For this review, use the dimensioned drawing (mm, ordinates from the lowest corner) and the shaded views. Coordinates: 2 decimals unless noted, no trailing zeros. Write each loop counter-clockwise with the first axis right and the second up, starting at its lowest first coordinate (ties: lowest second). Pieces come first, ordered by that corner, then holes.
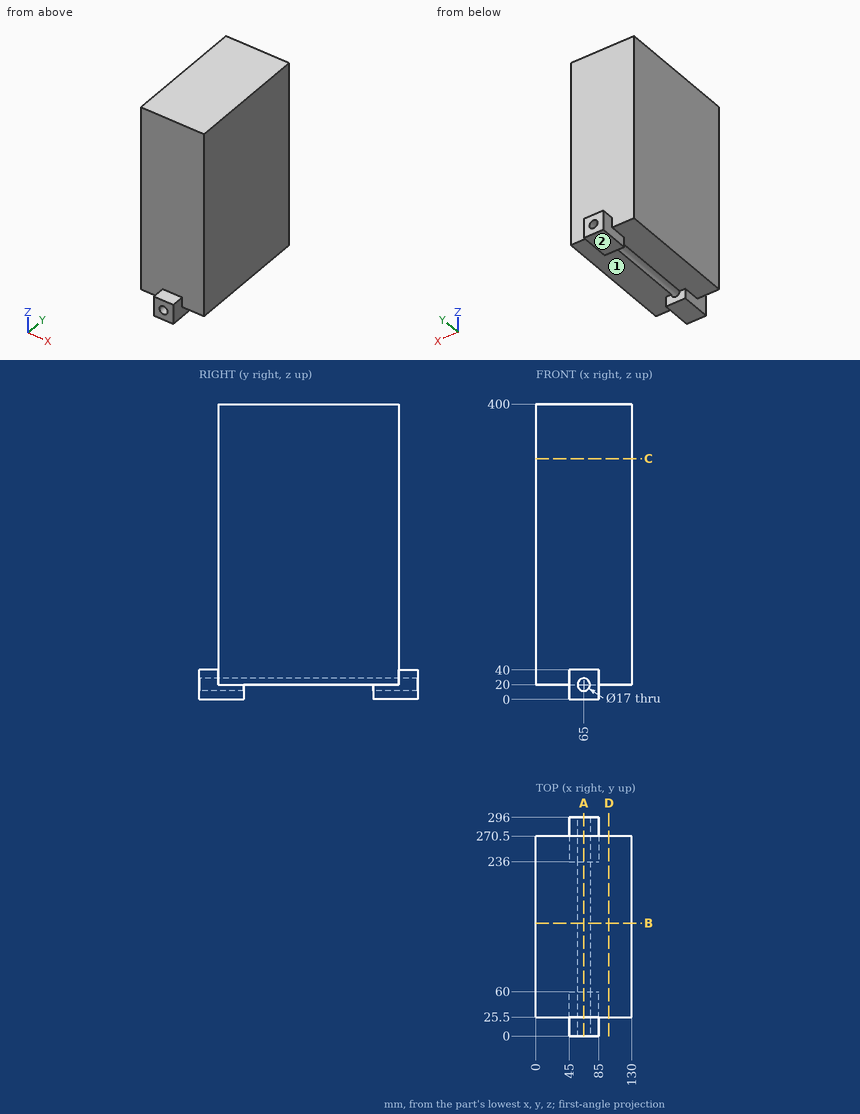
Item 1: Mouldability with a two-part tool opening along Y and no side actions: class the marked faces 1 and 2 as pulls with the +Y half, pulls with the -Y half, needs draft (parallel to the pull), parting line crosses it, or undercut.
Solved:
face 1: undercut
face 2: needs draft
Item 2: Take a section at C-C, the plane z = 326. Write out the cut boundary in (x, y), plus the area to 4 significant figures.
Solved:
outline: (0, 25.5) - (130, 25.5) - (130, 270.5) - (0, 270.5) - close
area: 31,850 mm2
Item 3: Take a section at D-D, the plane x = 99. Write out the cut boundary in (y, z).
Solved:
outline: (25.5, 20) - (270.5, 20) - (270.5, 400) - (25.5, 400) - close
Item 4: For pin 1 (1.5 mm diameter, centred on x = 100, z = 232.5, fed in from -Y); pin 2 (17 mm diameter, centred on x = 98.5, y = 208, fed in from -Z); pin 3 (13.5 mm diameter, centred on x = 65, z = 20, fed in from +Y); pin 4 (4 mm diameter, centred on x = 82.5, z = 300.5, fed in from +Y), all flat-tipped, find the tip position at first contact; note any pin that passes through.
Solved:
pin 1: stops at y = 25.5
pin 2: stops at z = 20
pin 3: passes through
pin 4: stops at y = 270.5
Item 5: Take a section at B-B, the plane y = 153. Write out the cut boundary in (x, z), plus the area to 3 significant figures.
Solved:
outline: (0, 20) - (56.5, 20) arc R8.5 cw to (73.5, 20) - (130, 20) - (130, 400) - (0, 400) - close
area: 49,300 mm2
Item 6: Take a section at A-A, the plane x = 65. Write out the cut boundary in (y, z).
Solved:
outline: (0, 0) - (60, 0) - (60, 11.5) - (0, 11.5) - close; (0, 28.5) - (296, 28.5) - (296, 40) - (270.5, 40) - (270.5, 400) - (25.5, 400) - (25.5, 40) - (0, 40) - close; (236, 0) - (296, 0) - (296, 11.5) - (236, 11.5) - close
Item 7: To check wall thickness, follow line 1 along X through (y, z) = (270, 19.5); line 2 along Y through (x, z) = (30.5, 104); line 3 along Z through (x, y) = (118, 164.5). State the ranges of each line that lie inside material, in increasing order.
Solved:
line 1: x = 45 to 56.51, 73.49 to 85
line 2: y = 25.5 to 270.5
line 3: z = 20 to 400
